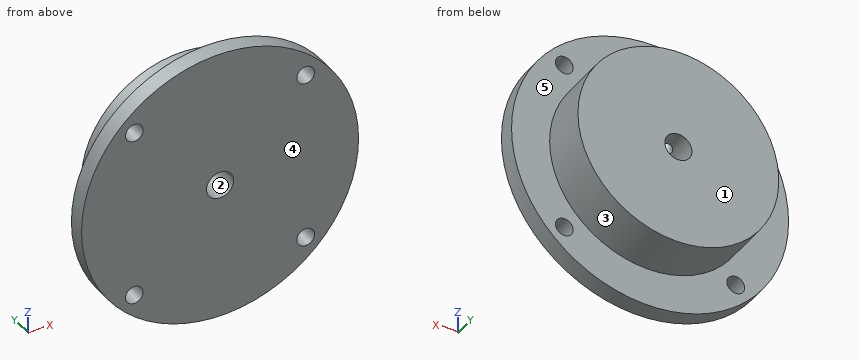
```python
from build123d import *

# Parameters (mm, degrees)
SKETCH10_R                 = 25.4
BOSS_EXTRUDE1_DEPTH        = 3.175
SKETCH13_R                 = 18.415
BOSS_EXTRUDE2_DEPTH        = 8.89
F_9_0_196_DIAMETER_HOLE1_D = 4.9784
SKETCH18_W                 = 1.35255
SKETCH18_H                 = 25.4
F_4_CLEARANCE_HOLE2_D      = 3.2639
F_4_CLEARANCE_HOLE2_DEPTH  = 3.302
F_4_CLEARANCE_HOLE2_TIP    = 0.980574487


with BuildPart() as part:
    # Sketch10 → Boss-Extrude1 (new body)
    with BuildSketch(Plane(origin=(0, 0, 0), x_dir=(1, 0, 0), z_dir=(0, 1, 0))):
        Circle(SKETCH10_R)
    extrude(amount=BOSS_EXTRUDE1_DEPTH)

    # Sketch13 → Boss-Extrude2 (add)
    with BuildSketch(Plane(origin=(0, 3.175, 0), x_dir=(1, 0, 0), z_dir=(0, 1, 0))):
        Circle(SKETCH13_R)
    extrude(amount=BOSS_EXTRUDE2_DEPTH)

    # #9 (0.196) Diameter Hole1 (through all)
    with Locations(Plane(origin=(0, 12.065, 0), x_dir=(1, 0, 0), z_dir=(0, 1, 0))):
        with Locations((0, 0)):
            Hole(F_9_0_196_DIAMETER_HOLE1_D / 2)

    # Sketch18 → #6-32 Tapped Hole2 (revolve, cut)
    with BuildSketch(Plane(origin=(0, 7.62, 0), x_dir=(0, 1, 0), z_dir=(1, 0, 0))):
        with Locations((0.676275, 12.7)):
            Rectangle(SKETCH18_W, SKETCH18_H)
    revolve(axis=Axis((0, 7.62, -6.35), (0, 0, 1)), mode=Mode.SUBTRACT)

    # #4 Clearance Hole2
    with Locations(Plane(origin=(0, 0, 0), x_dir=(-1, 0, 0), z_dir=(0, -1, 0))):
        with Locations((-15.715448212, -15.715448212), (15.715448212, -15.715448212), (15.715448212, 15.715448212), (-15.715448212, 15.715448212)):
            Hole(F_4_CLEARANCE_HOLE2_D / 2, depth=F_4_CLEARANCE_HOLE2_DEPTH)
            with Locations((0, 0, -(F_4_CLEARANCE_HOLE2_DEPTH + F_4_CLEARANCE_HOLE2_TIP / 2))):  # 118° drill point
                Cone(0, F_4_CLEARANCE_HOLE2_D / 2, F_4_CLEARANCE_HOLE2_TIP, mode=Mode.SUBTRACT)


solid = part.part
```
Geometry check sheet. Reference: the model listing, model coordinates, mm. Face numbers are marked on the shaded views. A direction names the side the tool comes from. Round coordinates to 2 decimals unless told otherwise and drop trailing zeros. Loops run counter-clockwise (first coordinate to the right, second up) from the corner with the lowest first, then second, coordinate; pieces in that order, holes last. Notation, with made-up numbers: (11, 75.25) - (20, 75.25) arc R15 ccw to (20, 86.25) - close; hole circle Ø6 at (41, 44.25). An arc over 180 degrees is marked (long way). Use a Markdown table: item, result.
Q1. Cross-section at C-C on y = 10.5. Record the cut outline in (x, z) (3 decimals), plus the area to 3 significant figures.
Solutions:
| item | result |
|---|---|
| outline | circle Ø36.83 at (0, 0); hole circle Ø4.978 at (0, 0) |
| area | 1,050 mm2 |
Q2. Cross-section at B-B on z = 0. Record the cut outline in (x, y) (3 decimals).
Solutions:
| item | result |
|---|---|
| outline | (-25.4, 0) - (-2.489, 0) - (-2.489, 12.065) - (-18.415, 12.065) - (-18.415, 3.175) - (-25.4, 3.175) - close; (2.489, 0) - (25.4, 0) - (25.4, 3.175) - (18.415, 3.175) - (18.415, 12.065) - (2.489, 12.065) - close |
Q3. Material ranges on line 1 (Z direction, x = -17, y = 0.75); line 2 (Y direction, x = 0, z = 5.75) (3 decimals); line 3 (X direction, y = 8.75, z = 0.5), recorded low to high.
Solutions:
| item | result |
|---|---|
| line 1 | z = -18.87 to -16.72, -14.71 to 14.71, 16.72 to 18.87 |
| line 2 | y = 0 to 6.267, 8.973 to 12.065 |
| line 3 | x = -18.41 to -2.44, 2.44 to 18.41 |
Q4. Cross-section at D-D on x = 8.5. Record the cut outline in (y, z) (3 decimals), plus the area to 3 significant figures.
Solutions:
| item | result |
|---|---|
| outline | (0, -23.936) - (3.175, -23.936) - (3.175, -16.336) - (12.065, -16.336) - (12.065, 16.336) - (3.175, 16.336) - (3.175, 23.936) - (0, 23.936) - close |
| area | 442 mm2 |
Q5. Draft check along Z on the marked faces 1, 2 and 3. Enter one of: released by +Z, released by -Z, zero draft, split by the parting line, or undercut.
Solutions:
| item | result |
|---|---|
| face 1 | zero draft |
| face 2 | undercut |
| face 3 | split by the parting line |
Q6. Go/stop test with flat-tipped pins: P1, Ø2, axis at x = -17.5, z = 9, coming from the -Y side; P2, Ø2, axis at x = 0, y = 7.62, coming from the +Z side; P3, Ø5, axis at x = -15.72, z = 15.72, coming from the +Y side (3 decimals). Record where each tip stops, or that it passes through.
Solutions:
| item | result |
|---|---|
| P1 | stops at y = 0 |
| P2 | stops at z = -2.28 |
| P3 | stops at y = 3.175 |
Q7. Access from +Z, -Z, +X, -X, +Y, -Y to the whole of each face (thin tool, end or side, straight path). Record for the marked faces 4 and 5.
Solutions:
| item | result |
|---|---|
| face 4 | +Z, -Z, +X, -X, -Y |
| face 5 | +Y |
Q8. Cross-section at A-A on x = 0. Record the cut outline in (y, z) (3 decimals), plus the area to 3 significant figures.
Solutions:
| item | result |
|---|---|
| outline | (0, -25.4) - (3.175, -25.4) - (3.175, -18.415) - (12.065, -18.415) - (12.065, -2.489) - (0, -2.489) - close; (0, 2.489) - (6.267, 2.489) - (6.267, 18.415) - (3.175, 18.415) - (3.175, 25.4) - (0, 25.4) - close; (8.973, 2.489) - (12.065, 2.489) - (12.065, 18.415) - (8.973, 18.415) - close |
| area | 386 mm2 |
